Part model, mm, in its own coordinate system. A direction names the side the tool comes from. Round coordinates to 2 decimals unless told otherwise and drop trailing zeros. Write each loop counter-clockwise with the first axis right and the second up, starting at its lowest first coordinate (ties: lowest second). Pieces come first, ordered by that corner, then holes.
1) Saw through at B-B on y = 7. Write the cut outline in (x, z).
2) Saw through at A-A on x = 215. Write the cut outline in (y, z), and give its area (3 significant figures).
3) Drill centre lines: L1, parallel to Z at x = 215, y = 8.6; L2, parallel to X at y = 6.5, z = 7; L3, parallel to Z at x = 231, y = 3.5. Where is each one in solid material? Low to high.
4) Pull direction Z, two halves, no side cores. Call faces 3 (the flat face through (145, 5, 10.9)), 4 (the flat face through (145, 6, -12.15)), 5 (the flat face through (295, 6, 0)): +Z half, -Z half, draft (parallel to the pull), parting line (faces both ways), or undercut.
5) Which spindle directions (+Z, -Z, +X, -X, +Y, -Y) get a long thin tool onto all of the face, cutting with end or side? Do faces 1 (the flat face through (145, 5, -10.9)), 2 (the flat face through (0, 6, 0)). Say none if no direction does.
6) Flat gauge pins, fed straight in: pin 1 (1.6 mm diameter, centred on x = 1, z = -3.5, fed in from -Y); pin 2 (3 mm diameter, centred on x = 37, z = 0, fed in from -Y). Where does each tip first touch, or does it go through?
Autodesk Inventor part; units mm, degrees
ref_plane "IP0_XY" through (0, 0, 0) normal (1, 0, 0) x (0, 0, -1)
ref_plane "IP0_YZ" through (0, 0, 0) normal (0, 0, -1) x (0, 1, 0)
ref_plane "IP0_ZX" through (0, 0, 0) normal (0, 1, 0) x (1, 0, 0)
sketch "Esquisse_1" plane through (0, 0, 0) normal (1, 0, 0) x (0, 1, 0)
  line L0 (2.6, 12.15) -> (2.6, 10.9)
  line L1 (2.6, 10.9) -> (8.25, 10.9)
  line L2 (8.25, 10.9) -> (8.25, -10.9)
  line L3 (8.25, -10.9) -> (2.6, -10.9)
  line L4 (2.6, -10.9) -> (2.6, -12.15)
  line L5 (2.6, -12.15) -> (9.5, -12.15)
  line L6 (9.5, -12.15) -> (9.5, 12.15)
  line L7 (9.5, 12.15) -> (2.6, 12.15)
extrude "Extrusion1" add sketch "Esquisse_1" along normal blind 295
sketch "Esquisse_2" plane through (0, 0, 0) normal (1, 0, 0) x (0, 1, 0)
  line L0 (9.5, 10.9) -> (3.5, 10.9)
  line L1 (3.5, 10.9) -> (3.5, -10.9)
  line L2 (3.5, -10.9) -> (9.5, -10.9)
  line L3 (9.5, -10.9) -> (9.5, 10.9)
extrude "Extrusion2" add sketch "Esquisse_2" along normal blind 1.5
sketch "Esquisse_3" plane through (295, 0, 0) normal (1, 0, 0) x (0, 0, -1)
  line L0 (-10.9, 9.5) -> (-10.9, 3.5)
  line L1 (-10.9, 3.5) -> (10.9, 3.5)
  line L2 (10.9, 3.5) -> (10.9, 9.5)
  line L3 (10.9, 9.5) -> (-10.9, 9.5)
extrude "Extrusion3" add sketch "Esquisse_3" against normal blind 1.5
sketch "Esquisse_4" plane through (0, 0, 0) normal (0, 1, 0) x (-1, 0, 0)
  circle A0 centre (-23.4, 0) radius 2.15
extrude "Extrusion4" cut sketch "Esquisse_4" along normal blind 9.5
sketch "Esquisse_5" plane through (0, 0, 0) normal (0, 1, 0) x (-1, 0, 0)
  arc A0 (-54.3, -2.15) -> (-54.3, 2.15) centre (-54.3, 0) ccw
  line L0 (-54.3, 2.15) -> (-56.5, 2.15)
  arc A1 (-56.5, 2.15) -> (-56.5, -2.15) centre (-56.5, 0) ccw
  line L1 (-56.5, -2.15) -> (-54.3, -2.15)
extrude "Extrusion5" cut sketch "Esquisse_5" along normal blind 9.5
sketch "Esquisse_6" plane through (0, 0, 0) normal (0, 1, 0) x (-1, 0, 0)
  arc A0 (-150.3, -2.15) -> (-150.3, 2.15) centre (-150.3, 0) ccw
  line L0 (-150.3, 2.15) -> (-152.5, 2.15)
  arc A1 (-152.5, 2.15) -> (-152.5, -2.15) centre (-152.5, 0) ccw
  line L1 (-152.5, -2.15) -> (-150.3, -2.15)
extrude "Extrusion6" cut sketch "Esquisse_6" along normal blind 9.5
sketch "Esquisse_7" plane through (0, 0, 0) normal (0, 1, 0) x (-1, 0, 0)
  arc A0 (-182.3, -2.15) -> (-182.3, 2.15) centre (-182.3, 0) ccw
  line L0 (-182.3, 2.15) -> (-184.5, 2.15)
  arc A1 (-184.5, 2.15) -> (-184.5, -2.15) centre (-184.5, 0) ccw
  line L1 (-184.5, -2.15) -> (-182.3, -2.15)
extrude "Extrusion7" cut sketch "Esquisse_7" along normal blind 9.5
sketch "Esquisse_8" plane through (0, 0, 0) normal (0, 1, 0) x (-1, 0, 0)
  arc A0 (-246.3, -2.15) -> (-246.3, 2.15) centre (-246.3, 0) ccw
  line L0 (-246.3, 2.15) -> (-248.5, 2.15)
  arc A1 (-248.5, 2.15) -> (-248.5, -2.15) centre (-248.5, 0) ccw
  line L1 (-248.5, -2.15) -> (-246.3, -2.15)
extrude "Extrusion8" cut sketch "Esquisse_8" along normal blind 9.5
sketch "Esquisse_9" plane through (0, 0, 0) normal (0, 1, 0) x (-1, 0, 0)
  arc A0 (-278.3, -2.15) -> (-278.3, 2.15) centre (-278.3, 0) ccw
  line L0 (-278.3, 2.15) -> (-280.5, 2.15)
  arc A1 (-280.5, 2.15) -> (-280.5, -2.15) centre (-280.5, 0) ccw
  line L1 (-280.5, -2.15) -> (-278.3, -2.15)
extrude "Extrusion9" cut sketch "Esquisse_9" along normal blind 9.5
sketch "Esquisse_10" plane through (0, 0, 0) normal (0, 1, 0) x (-1, 0, 0)
  circle A0 centre (-87.5, 0) radius 5
extrude "Extrusion10" cut sketch "Esquisse_10" along normal blind 9.5
sketch "Esquisse_11" plane through (0, 0, 0) normal (0, 1, 0) x (-1, 0, 0)
  circle A0 centre (-215, 0) radius 5
extrude "Extrusion11" cut sketch "Esquisse_11" along normal blind 9.5
ref_plane "IP0_XY" through (0, 0, 0) normal (1, 0, 0) x (0, 0, -1)
ref_plane "IP0_YZ" through (0, 0, 0) normal (0, 0, -1) x (0, 1, 0)
ref_plane "IP0_ZX" through (0, 0, 0) normal (0, 1, 0) x (1, 0, 0)
properties part number "MICHAUD CHAILLY B3 - 21 - 30 - 2"
Completed:
1. outline: (0, -12.15) - (295, -12.15) - (295, 12.15) - (0, 12.15) - close; hole (1.5, -10.9) - (293.5, -10.9) - (293.5, 10.9) - (1.5, 10.9) - close
2. outline: (2.6, -12.15) - (9.5, -12.15) - (9.5, -5) - (8.25, -5) - (8.25, -10.9) - (2.6, -10.9) - close; (2.6, 10.9) - (8.25, 10.9) - (8.25, 5) - (9.5, 5) - (9.5, 12.15) - (2.6, 12.15) - close
2. area: 32.0 mm2
3. L1: z = -12.15 to -5, 5 to 12.15
3. L2: x = 0 to 1.5, 293.5 to 295
3. L3: z = -12.15 to -10.9, 10.9 to 12.15
4. face 3: undercut
4. face 4: -Z half
4. face 5: draft
5. face 1: -Y
5. face 2: +Z, -Z, -X, +Y, -Y
6. pin 1: stops at y = 3.5
6. pin 2: stops at y = 8.25
